For this review, take the finished solid that the model builds, in its own axes (mm). Give positions to 0.01 mm unless a question says otherwise; leave off trailing zeros. Write each loop counter-clockwise with the first axis right and the second up, starting at its lowest first coordinate (ties: lowest second). Pieces come first, ordered by that corner, then holes. Notation, with made-up numbers: M 23.5,-17 L 28.5,-17 A19 ccw 28.5,12 Z; hole C -15.75,61.25 d11. An arc over 180 degrees is marked long. Use one line per item in the form item = value. Start each with the question number.
Q1. Consider section D-D on y = 10. Write out the cut boundary in (x, z) (3 decimals).
Q2. Consider section C-C on z = 2.35. Write out the cut boundary in (x, y).
Q3. Consider section A-A on x = 0. Write out the cut boundary in (y, z) (3 decimals).
Q4. Mouldability with a two-part tool opening along Y and no side actions: class faces 1 (the cylindrical face through (-14.43, -14.4, 1.61)), 2 (the cylindrical face through (-14.4, 14.43, 1.61)), 3 (the flat face through (15, 0, 2)), 4 (the cylindrical face through (11.464, 10.761, 1.61)) as released by +Y, released by -Y, zero draft, split by the parting line, or undercut.
Q5. For probe 1 along X at (y, z) = (10, 1.2); probe 2 along Y at (x, z) = (8.5, 0.45), list the stretches that pass through material, from the lowest coordinate up. Write a range as [from, to].
Autodesk Inventor part; units mm, degrees
ref_plane "YZ Plane" through (0, 0, 0) normal (1, 0, 0) x (0, 1, 0)
ref_plane "XZ Plane" through (0, 0, 0) normal (0, 1, 0) x (-1, 0, 0)
ref_plane "XY Plane" through (0, 0, 0) normal (0, 0, 1) x (1, 0, 0)
sketch "Sketch1" plane through (0, 0, 0) normal (0, 0, 1) x (1, 0, 0)
  line L0 (10, -10) -> (-10, -10) construction
  line L1 (-10, -10) -> (-10, 10) construction
  line L2 (-10, 10) -> (10, 10) construction
  line L3 (10, 10) -> (10, -10) construction
  line L4 (10, -10) -> (-10, 10) construction
  line L5 (-10, -10) -> (10, 10) construction
  line L6 (15, -15) -> (-15, -15)
  line L7 (-15, -15) -> (-15, 15)
  line L8 (-15, 15) -> (15, 15)
  line L9 (15, 15) -> (15, -15)
  line L10 (15, -15) -> (-15, 15) construction
  line L11 (-15, -15) -> (15, 15) construction
  point P0 (0, 0)
  point P1 (0, 0)
  dimension "d0" = 20
  dimension "d1" = 20
  dimension "d2" = 30
  dimension "d3" = 30
extrude "Extrusion1" add sketch "Sketch1" along normal blind 3.175
fillet "Fillet1" radius 2 4 edges at (-15, 15, 1.5875) (-15, -15, 1.5875) (15, -15, 1.5875) (15, 15, 1.5875)
hole "Hole1" at (-10, 10, 0) at (10, 10, 0) at (10, -10, 0) at (-10, -10, 0) direction (0, 0, 1) diameter 3.3 end through all
hole "Hole2" at (0, 0, 0) direction (0, 0, 1) diameter 6.3 end through all
equation "\"d3\" = d2"
properties part number "Inductive Sensor Plate" material "Aluminum 6061"
Working result:
q1.outline = M -15,0 L -11.65,0 L -11.65,3.175 L -15,3.175 Z; M -8.35,0 L 8.35,0 L 8.35,3.175 L -8.35,3.175 Z; M 11.65,0 L 15,0 L 15,3.175 L 11.65,3.175 Z
q2.outline = M -15,-13 A2 ccw -13,-15 L 13,-15 A2 ccw 15,-13 L 15,13 A2 ccw 13,15 L -13,15 A2 ccw -15,13 Z; hole C -10,-10 d3.3; hole C -10,10 d3.3; hole C 0,0 d6.3; hole C 10,-10 d3.3; hole C 10,10 d3.3
q3.outline = M -15,0 L -3.15,0 L -3.15,3.175 L -15,3.175 Z; M 3.15,0 L 15,0 L 15,3.175 L 3.15,3.175 Z
q4.face_1 = released by -Y
q4.face_2 = released by +Y
q4.face_3 = zero draft
q4.face_4 = undercut
q5.probe_1 = [-15, -11.65], [-8.35, 8.35], [11.65, 15]
q5.probe_2 = [-15, -10.69], [-9.31, 9.31], [10.69, 15]
